For this review, take the finished solid that the model builds, in its own axes (mm). Face numbers are marked on the shaded views. Round coordinates to 2 decimals unless told otherwise and drop trailing zeros. Write each loop counter-clockwise with the first axis right and the second up, starting at its lowest first coordinate (ties: lowest second). Pieces come first, ordered by that corner, then holes. Notation, with made-up numbers: (38.5, 75.25) -> (85.5, 75.25) arc R7 cw to (85.5, 81.25) -> close; hole circle Ø3 at (-37, 56). An arc over 180 degrees is marked (long way). Answer in a Markdown table with one row per item.
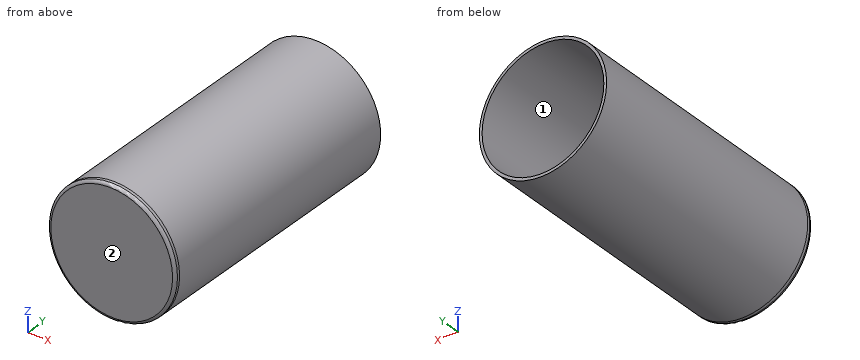
Autodesk Inventor part; units mm, degrees
ref_plane "YZ Plane" through (0, 0, 0) normal (1, 0, 0) x (0, 1, 0)
ref_plane "XZ Plane" through (0, 0, 0) normal (0, 1, 0) x (-1, 0, 0)
ref_plane "XY Plane" through (0, 0, 0) normal (0, 0, 1) x (1, 0, 0)
sketch "Sketch1" plane through (0, 0, 0) normal (0, 1, 0) x (-1, 0, 0)
  circle A0 centre (0, 0) radius 22
  circle A1 centre (0, 0) radius 23
  dimension "d0" = 44
  dimension "d1" = 46
extrude "Extrusion1" add sketch "Sketch1" along normal blind 95
sketch "Sketch2" plane through (0, 0, 0) normal (0, -1, 0) x (1, 0, 0)
  circle A0 centre (0, 0) radius 23
  circle A1 centre (0, -23) radius 0.5
  dimension "d8" = 1
sketch "Sketch3" plane through (0, 0, 0) normal (0, -1, 0) x (1, 0, 0)
  circle A0 centre (0, 0) radius 23
  dimension "d4" = 46
extrude "Extrusion2" add sketch "Sketch3" along normal blind 2
fillet "Fillet1" radius 1 1 edges at (-23, -2, 0)
properties part number "Dalek Light"
1) For line 1 (Z direction, x = 0, y = 55); line 2 (Y direction, x = 1, z = -10); line 3 (X direction, y = 12.5, z = 15.5), list the stretches that pass through material, from the lowest coordinate up. Write a range as [from, to].
Solved:
| item | result |
|---|---|
| line 1 | [-23, -22], [22, 23] |
| line 2 | [-2, 0] |
| line 3 | [-16.99, -15.61], [15.61, 16.99] |
2) Consider section B-B on z = 0. State the section outline as (x, y) points.
Solved:
| item | result |
|---|---|
| outline | (-23, -1) arc R1 ccw to (-22, -2) -> (22, -2) arc R1 ccw to (23, -1) -> (23, 95) -> (22, 95) -> (22, 0) -> (-22, 0) -> (-22, 95) -> (-23, 95) -> close |
3) Mouldability with a two-part tool opening along Z and no side actions: class the marked faces 1 and 2 as pulls with the +Z half, pulls with the -Z half, needs draft (parallel to the pull), parting line crosses it, or undercut.
Solved:
| item | result |
|---|---|
| face 1 | undercut |
| face 2 | needs draft |
4) Clearance check with flat-ended pins moving along their axes: pin 1 Ø1.5 at (x, y) = (6, 76.5) entering from +Z; pin 2 Ø8 at (y, z) = (68.5, -16) entering from +X; pin 3 Ø3 at (x, y) = (11, 56) entering from +Z. State where each tip first meets the part, or that it passes through.
Solved:
| item | result |
|---|---|
| pin 1 | z = 22.39 |
| pin 2 | x = 19.62 |
| pin 3 | z = 20.95 |
5) Consider section A-A on x = 0. State the section outline as (y, z) points, then the cut area to 3 significant figures.
Solved:
| item | result |
|---|---|
| outline | (-2, -22) arc R1 ccw to (-1, -23) -> (95, -23) -> (95, -22) -> (0, -22) -> (0, 22) -> (95, 22) -> (95, 23) -> (-1, 23) arc R1 ccw to (-2, 22) -> close |
| area | 282 mm² |
6) Consider section C-C on y = 59. State the section outline as (x, z) points.
Solved:
| item | result |
|---|---|
| outline | circle Ø46 at (0, 0); hole circle Ø44 at (0, 0) |
